For this review, take the finished solid that the model builds, in its own axes (mm). Face numbers are marked on the shaded views. A direction names the side the tool comes from. Give positions to 0.01 mm unless a question says otherwise; leave off trailing zeros. Order: outer loops, then holes, each group sorted by start corner. A loop starts at its lowest first (then second) coordinate and runs counter-clockwise, first axis right, second up. Notation, with made-up numbers: M -32,30 L -15,30 A15 cw -15,46 Z; hole C -3.5,41.25 d8. An arc over 180 degrees is marked long. Answer as CSV lines item,"result". Start each with the question number.
1. We need section D-D, the plane y = -15. Give the boundary of the cut face in (x, z), and give its area (3 significant figures).
2. Clearance check with flat-ended pins moving along their axes: P1, Ø12, axis at y = -3, z = 34, coming from the -X side; P2, Ø11, axis at x = -35.5, z = 25.5, coming from the -Y side; P3, Ø5, axis at x = 33, z = 26.5, coming from the +Y side; P4, Ø12, axis at x = 0, y = 0, coming from the +Z side. State where each tip first meets the part, or that it passes through.
3. Machinability: for the marked faces 1, 2, 3 and 4, which of the approach directions +Z, -Z, +X, -X, +Y, -Y give a long, thin tool a straight path to every point of the face, cutting with its end or side? Answer none if there is none.
4. We need section A-A, the plane z = 44.5. Give the boundary of the cut face in (x, y).
5. For line 1 along X through (y, z) = (-28, 22); line 2 along Y through (x, z) = (0, 3); line 3 along Z through (x, y) = (45.5, -6), list the stretches that pass through material, from the lowest coordinate up.
6. Mouldability with a two-part tool opening along Y and no side actions: class the marked faces 5, 6 and 7 as pulls with the +Y half, pulls with the -Y half, needs draft (parallel to the pull), parting line crosses it, or undercut.
7. We need section B-B, the plane x = 0. Give the boundary of the cut face in (y, z).
8. We need section C-C, the plane y = 0. Give the boundary of the cut face in (x, z).
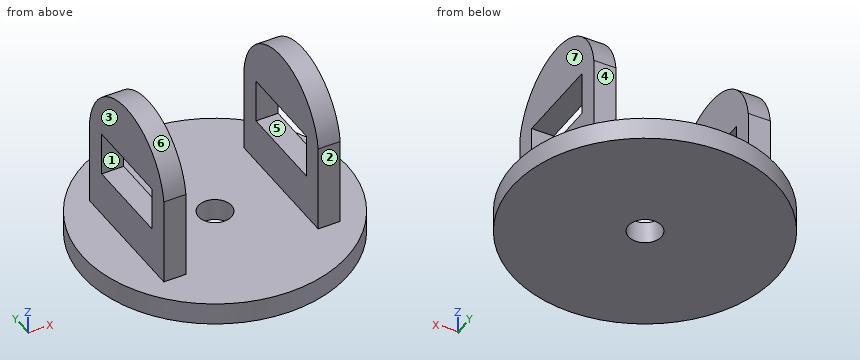
from build123d import *

# Parameters (mm, degrees)
SKETCH_1_R          = 60
EXTRUDE_1_DEPTH     = 10
SKETCH_3_W          = 19.9
SKETCH_3_H          = 40.7
EXTRUDE_4_DEPTH     = 10
SKETCH_10_W         = 19.9
SKETCH_10_H         = 40.7
EXTRUDE_7_DEPTH     = 10
SKETCH_11_R         = 7.5
CUT_EXTRUDE_1_DEPTH = 108.636941111


with BuildPart() as part:
    # 스케치1 → 보스-돌출1 (new body)
    with BuildSketch(Plane.XY):
        Circle(SKETCH_1_R)
    extrude(amount=EXTRUDE_1_DEPTH)

    # 스케치3 → 보스-돌출4 (add)
    with BuildSketch(Plane(origin=(30, 0, 0), x_dir=(0, 0, -1), z_dir=(1, 0, 0))):
        with BuildLine():
            Line((-10, 0), (-10, 30.023943052))
            Line((-10, 30.023943052), (-50, 30.023943052))
            ThreePointArc((-50, 30.023943052), (-76.224701523, 0.023943052), (-50, -29.976056948))
            Line((-50, -29.976056948), (-10, -29.976056948))
            Line((-10, -29.976056948), (-10, 0))
        make_face()
        with Locations((-40, 0)):
            Rectangle(SKETCH_3_W, SKETCH_3_H, mode=Mode.SUBTRACT)
    extrude(amount=EXTRUDE_4_DEPTH)

    # 스케치10 → 보스-돌출7 (add)
    with BuildSketch(Plane(origin=(-40, 0, 0), x_dir=(0, 0, -1), z_dir=(1, 0, 0))):
        with BuildLine():
            Line((-10, 30.023943052), (-50, 30.023943052))
            ThreePointArc((-50, 30.023943052), (-76.224701523, 0.023943052), (-50, -29.976056948))
            Line((-50, -29.976056948), (-10, -29.976056948))
            Line((-10, -29.976056948), (-10, 30.023943052))
        make_face()
        with Locations((-40, 0)):
            Rectangle(SKETCH_10_W, SKETCH_10_H, mode=Mode.SUBTRACT)
    extrude(amount=EXTRUDE_7_DEPTH)

    # 스케치11 → 컷-돌출1 (cut, through all)
    with BuildSketch(Plane.XY.offset(10)):
        Circle(SKETCH_11_R)
    extrude(amount=-CUT_EXTRUDE_1_DEPTH, mode=Mode.SUBTRACT)


solid = part.part
Result set:
1,outline,"M -58.09,0 L 58.09,0 L 58.09,10 L 40,10 L 40,30.05 L 30,30.05 L 30,10 L -30,10 L -30,30.05 L -40,30.05 L -40,10 L -58.09,10 Z; M -40,49.95 L -30,49.95 L -30,72.23 L -40,72.23 Z; M 30,49.95 L 40,49.95 L 40,72.23 L 30,72.23 Z"
1,area,"2,010 mm2"
2,P1,"x = -40"
2,P2,"y = -29.98"
2,P3,"y = 30.02"
2,P4,"through"
3,face 1,"+X, -X"
3,face 2,"+Z, +X, -X, -Y"
3,face 3,"+Z, -X, +Y, -Y"
3,face 4,"+Z, +X, -X, +Y"
4,outline,"M -40,-29.98 L -30,-29.98 L -30,-20.35 L -40,-20.35 Z; M -40,20.35 L -30,20.35 L -30,30.02 L -40,30.02 Z; M 30,-29.98 L 40,-29.98 L 40,-20.35 L 30,-20.35 Z; M 30,20.35 L 40,20.35 L 40,30.02 L 30,30.02 Z"
5,line 1,"-40 to -30, 30 to 40"
5,line 2,"-60 to -7.5, 7.5 to 60"
5,line 3,"0 to 10"
6,face 5,"undercut"
6,face 6,"parting line crosses it"
6,face 7,"needs draft"
7,outline,"M -60,0 L -7.5,0 L -7.5,10 L -60,10 Z; M 7.5,0 L 60,0 L 60,10 L 7.5,10 Z"
8,outline,"M -60,0 L -7.5,0 L -7.5,10 L -30,10 L -30,30.05 L -40,30.05 L -40,10 L -60,10 Z; M -40,49.95 L -30,49.95 L -30,76.22 L -40,76.22 Z; M 7.5,0 L 60,0 L 60,10 L 40,10 L 40,30.05 L 30,30.05 L 30,10 L 7.5,10 Z; M 30,49.95 L 40,49.95 L 40,76.22 L 30,76.22 Z"
